```python
from build123d import *

# Parameters (mm, degrees)
SKETCH001_W       = 20
SKETCH001_H       = 20
PAD_DEPTH         = 10
SKETCH003_R       = 1.6
POCKET_DEPTH      = 0.001
POCKET_DEPTH_BACK = 10.001
SKETCH002_R       = 3.5
POCKET001_DEPTH   = 3
POCKET002_DEPTH   = 0.2
SKETCH005_W       = 3.2
SKETCH005_H       = 3.2
POCKET003_DEPTH   = 0.2
SKETCH006_W       = 6
SKETCH006_H       = 5
PAD001_DEPTH      = 1
PAD001_TAPER      = 45
PAD001_FACE19_W   = 20
PAD001_FACE19_H   = 10
PAD002_DEPTH      = 0.1


with BuildPart() as part:
    # Sketch001 → Pad (new body)
    with BuildSketch(Plane.XY):
        Rectangle(SKETCH001_W, SKETCH001_H)
    extrude(amount=PAD_DEPTH)

    # Sketch003 → Pocket (cut, two sides)
    with BuildSketch(Plane.XY) as pocket_sk:
        Circle(SKETCH003_R)
    extrude(amount=-POCKET_DEPTH, mode=Mode.SUBTRACT)
    extrude(pocket_sk.sketch, amount=POCKET_DEPTH_BACK, mode=Mode.SUBTRACT)

    # Sketch002 → Pocket001 (cut)
    with BuildSketch(Plane.XY):
        Circle(SKETCH002_R)
    extrude(amount=POCKET001_DEPTH, mode=Mode.SUBTRACT)

    # Sketch004 (on Face9 of Pocket001) → Pocket002 (cut)
    with BuildSketch(Plane(origin=(0, 0, 3), x_dir=(1, 0, 0), z_dir=(0, 0, -1))):
        with BuildLine():
            ThreePointArc((1.6, 3.1128764833), (0, 3.5), (-1.6, 3.1128764833))
            Line((-1.6, 3.1128764833), (-1.6, -3.1128764833))
            ThreePointArc((-1.6, -3.1128764833), (0, -3.5), (1.6, -3.1128764833))
            Line((1.6, 3.1128764833), (1.6, -3.1128764833))
        make_face()
    extrude(amount=-POCKET002_DEPTH, mode=Mode.SUBTRACT)

    # Sketch005 (on Face13 of Pocket002) → Pocket003 (cut)
    with BuildSketch(Plane(origin=(0, 0, 3.2), x_dir=(1, 0, 0), z_dir=(0, 0, -1))):
        Rectangle(SKETCH005_W, SKETCH005_H)
    extrude(amount=-POCKET003_DEPTH, mode=Mode.SUBTRACT)

    # Sketch006 (on Face11 of Pocket003) → Pad001 (join)
    with BuildSketch(Plane.XY.offset(10)):
        with Locations((0, 5.5)):
            Rectangle(SKETCH006_W, SKETCH006_H)
        with Locations((0, -5.5)):
            Rectangle(SKETCH006_W, SKETCH006_H)
    extrude(amount=PAD001_DEPTH, taper=PAD001_TAPER)

    # Pad001 Face19 → Pad002 (add)
    with BuildSketch(Plane(origin=(10, 0, 5), x_dir=(0, -1, 0), z_dir=(1, 0, 0))):
        Rectangle(PAD001_FACE19_W, PAD001_FACE19_H)
    extrude(amount=PAD002_DEPTH)


solid = part.part
```
The model under review builds one solid part; all positions refer to its coordinate system, in mm. A direction names the side the tool comes from. Round coordinates to 2 decimals unless told otherwise and drop trailing zeros. Loops run counter-clockwise (first coordinate to the right, second up) from the corner with the lowest first, then second, coordinate; pieces in that order, holes last. Notation, with made-up numbers: (-22, -39.5) - (23, -39.5) arc R24 ccw to (23, -2.5) - close; hole circle Ø1 at (52, 68.25). An arc over 180 degrees is marked (long way). Use a Markdown table: item, result. Add a question column.
Q1. Add section D-D (x = -2.5). State the section outline as (y, z) points, plus the area to 3 significant figures.
Q2. Add section C-C (y = 1). State the section outline as (x, z) points, plus the area to 3 significant figures.
Q3. Add section B-B (y = 7.5). State the section outline as (x, z) points, plus the area to 3 significant figures.
Q4. Machinability: for faces 4 (the face through (10.1, 0, 5)), 5 (the face through (2, 0, 3)), 6 (the face through (0, 3.5, 10.5)), 7 (the face through (0, -2, 10)), which of the approach directions +Z, -Z, +X, -X, +Y, -Y give a long, thin tool a straight path to every point of the face, cutting with its end or side? Answer none if there is none.
Q5. For probe 1 along Y at (x, z) = (0, 7.5); probe 2 along Y at (x, z) = (0, 1.8); probe 3 along X at (y, z) = (0, 2), list the stretches that pass through material, from the lowest coordinate up.
Q6. Add section A-A (z = 4.75). State the section outline as (x, y) points, plus the area to 3 significant figures.
Q7. Insertion check: pin 1 Ø4 at (x, y) = (0, 0) entering from -Z; pin 2 Ø3 at (x, y) = (-5, -0.5) entering from +Z; pin 3 Ø1.8 at (x, y) = (0.5, -1) entering from -Z. Each pin has a flat end and moves straight along its axis. Give the tip position at first contact, or say it passes through.
Q8. The part is to be moulded in two halves that separate along X. For faces 1 (the face through (0, -10, 5)), 2 (the face through (2.5, -5.5, 10.5)), 3 (the face through (-1.3, 1.2, 3.4)), say which applies: pulls with the +X half, pulls with the -X half, needs draft (parallel to the pull), parting line crosses it, or undercut.
Worked answers:
| question | item | result |
|---|---|---|
| 1 | outline | (-10, 0) - (-2.45, 0) - (-2.45, 3) - (2.45, 3) - (2.45, 0) - (10, 0) - (10, 10) - (8, 10) - (7.5, 10.5) - (3.5, 10.5) - (3, 10) - (-3, 10) - (-3.5, 10.5) - (-7.5, 10.5) - (-8, 10) - (-10, 10) - close |
| 1 | area | 190 mm² |
| 2 | outline | (-10, 0) - (-3.35, 0) - (-3.35, 3) - (-1.6, 3) - (-1.6, 3.4) - (-1.25, 3.4) - (-1.25, 10) - (-10, 10) - close; (1.25, 3.4) - (1.6, 3.4) - (1.6, 3) - (3.35, 3) - (3.35, 0) - (10.1, 0) - (10.1, 10) - (1.25, 10) - close |
| 2 | area | 163 mm² |
| 3 | outline | (-10, 0) - (10.1, 0) - (10.1, 10) - (3, 10) - (2.5, 10.5) - (-2.5, 10.5) - (-3, 10) - (-10, 10) - close |
| 3 | area | 204 mm² |
| 4 | face 4 | +Z, -Z, +X, +Y, -Y |
| 4 | face 5 | -Z |
| 4 | face 6 | +Z, +X, -X |
| 4 | face 7 | +Z |
| 5 | probe 1 | -10 to -1.6, 1.6 to 10 |
| 5 | probe 2 | -10 to -3.5, 3.5 to 10 |
| 5 | probe 3 | -10 to -3.5, 3.5 to 10.1 |
| 6 | outline | (-10, -10) - (10.1, -10) - (10.1, 10) - (-10, 10) - close; hole circle Ø3.2 at (0, 0) |
| 6 | area | 394 mm² |
| 7 | pin 1 | z = 3 |
| 7 | pin 2 | z = 10 |
| 7 | pin 3 | z = 3.2 |
| 8 | face 1 | needs draft |
| 8 | face 2 | pulls with the +X half |
| 8 | face 3 | undercut |
